from build123d import *

# Parameters (mm, degrees)
SKETCH1_R           = 12.578
SKETCH1_R_2         = 9.398
BOSS_EXTRUDE1_DEPTH = 3.175
FILLET1_R           = 38.1
FILLET2_R           = 6.35


with BuildPart() as part:
    # Sketch1 → Boss-Extrude1 (new, symmetric)
    # profile 1 of 4: a face of its own
    with BuildSketch(Plane.XY):
        with BuildLine():
            Line((550.906377784, 50.55819174), (568.724608053, 41.896435909))
            ThreePointArc((568.724608053, 41.896435909), (571.307203408, 34.427721881), (563.838489379, 31.845126527))
            Line((563.838489379, 31.845126527), (546.02025911, 40.506882357))
            Line((546.02025911, 40.506882357), (543.244055318, 34.795911117))
            Line((543.244055318, 34.795911117), (602.068897859, 6.200118203))
            Line((602.068897859, 6.200118203), (619.322536705, 15.354662769))
            ThreePointArc((619.322536705, 15.354662769), (624.245533427, 18.531839743), (630.07371037, 19.134088663))
            Line((630.07371037, 19.134088663), (553.682581576, 56.26916298))
            Line((553.682581576, 56.26916298), (550.906377784, 50.55819174))
        make_face()
    # profile 2 of 4: a face of its own
    with BuildSketch(Plane.XY):
        with BuildLine():
            ThreePointArc((619.635184113, -2.3391632), (615.840878926, 6.443467165), (619.322536705, 15.354662769))
            Line((619.322536705, 15.354662769), (602.068897859, 6.200118203))
            Line((602.068897859, 6.200118203), (619.635184113, -2.3391632))
        make_face()
    # profile 3 of 4: a face of its own
    with BuildSketch(Plane.XY):
        with Locations((628.416915809, 6.665683962)):
            Circle(SKETCH1_R)
        with Locations((628.416915809, 6.665683962)):
            Circle(SKETCH1_R_2, mode=Mode.SUBTRACT)
    # profile 4 of 4: a face of its own
    with BuildSketch(Plane.XY):
        with BuildLine():
            Line((619.635184113, -2.3391632), (602.068897859, 6.200118203))
            Line((602.068897859, 6.200118203), (544.291028723, -24.456028169))
            Line((544.291028723, -24.456028169), (547.267260579, -30.065354683))
            Line((547.267260579, -30.065354683), (564.768359303, -20.779511294))
            ThreePointArc((564.768359303, -20.779511294), (572.323650668, -23.096634594), (570.006527369, -30.651925959))
            Line((570.006527369, -30.651925959), (552.505428645, -39.937769348))
            Line((552.505428645, -39.937769348), (555.4816605, -45.547095862))
            Line((555.4816605, -45.547095862), (630.513168482, -5.736404924))
            ThreePointArc((630.513168482, -5.736404924), (624.667353131, -5.3404338), (619.635184113, -2.3391632))
        make_face()
    extrude(amount=BOSS_EXTRUDE1_DEPTH, both=True)

    # Fillet1
    # the kernel refuses this fillet: 38.1 mm, written as the material it adds along each edge
    with BuildSketch(Plane(origin=(602.068897859, 6.200118203, -3.175), x_dir=(-0.8993655496308585, 0.43719744754193623, 0), z_dir=(0, 0, 1))) as fillet1_piece_1:
        with BuildLine():
            CenterArc((73.33595186, 37.265834599), FILLET1_R, 155.886500773, 102.102011478)
            Line((38.560636086, 52.831418843), (0, 0))
            Line((0, 0), (65.407044516, 0))
        make_face()
    extrude(amount=6.35)

    # Fillet2
    fillet2_edges = [part.edges().sort_by_distance(p)[0] for p in [
        (630.07371037, 19.134088663, 0),
        (630.513168482, -5.736404924, 0),
    ]]
    fillet(fillet2_edges, radius=FILLET2_R)


solid = part.part
Geometry check sheet. Reference: the model listing, model coordinates, mm. A direction names the side the tool comes from. Give positions to 0.01 mm unless a question says otherwise; leave off trailing zeros. Loops run counter-clockwise (first coordinate to the right, second up) from the corner with the lowest first, then second, coordinate; pieces in that order, holes last. Notation, with made-up numbers: (-36, -21) -> (8, -21) arc R32 ccw to (8, 14) -> close; hole circle Ø11 at (-9.75, -32). An arc over 180 degrees is marked (long way). Answer in a Markdown table with one row per item. Add a question column.
1) Gauge pin test, flat ends, axial feed: P1, Ø1.5, axis at x = 591.5, z = 0.5, coming from the +Y side; P2, Ø1.5, axis at x = 565.5, z = 2, coming from the -Y side; P3, Ø3, axis at x = 573, z = -2, coming from the -Y side. Record the tip position at first contact, or that the pin passes through.
2) Set-up check for faces 4 (the face through (583, 2, 3.175)), 5 (the face through (555.054, 36.115, 0.044)), 6 (the face through (559.69, 46.29, 0.04)): record each of +Z, -Z, +X, -X, +Y, -Y from which the full face is reachable in a straight line by a thin tool's end or side.
3) Cross-section at C-C on z = -1.5. Record the boundary of the cut face in (x, y).
4) Material ranges on probe 1 along Y at (x, z) = (569.5, -1.75); probe 2 along Y at (x, z) = (566.5, -2.75); probe 3 along Y at (x, z) = (628.5, -0.75), recorded low to high. Write a range as from..to.
5) Cross-section at B-B on y = -27. Record the boundary of the cut face in (x, z) (3 decimals).
6) Cross-section at A-A on x = 621. Record the boundary of the cut face in (y, z) (3 decimals).
7) Draft check along Y on faces 1 (the face through (561.38, -35.23, 0.04)), 2 (the face through (553.97, -42.7, 0.04)), 3 (the face through (544.65, 37.69, 0.04)). Enter one of: pulls with the +Y half, pulls with the -Y half, needs draft (parallel to the pull), parting line crosses it, or undercut.
8) Cross-section at D-D on x = 593. Record the boundary of the cut face in (y, z) (3 decimals).
Outcome:
| question | item | result |
|---|---|---|
| 1 | P1 | stops at y = 38.25 |
| 1 | P2 | stops at y = -40.63 |
| 1 | P3 | stops at y = -37.05 |
| 2 | face 4 | +Z, +X, -X, +Y, -Y |
| 2 | face 5 | +Z, -Z |
| 2 | face 6 | +Z, -Z, -X |
| 3 | outline | (543.24, 34.8) arc R38.1 cw to (544.29, -24.46) -> (547.27, -30.07) -> (564.77, -20.78) arc R5.59 cw to (570.01, -30.65) -> (552.51, -39.94) -> (555.48, -45.55) -> (629.7, -6.17) arc R6.35 cw to (631.25, -5.59) arc R12.58 ccw to (630.81, 19.01) arc R6.35 cw to (629.25, 19.54) -> (553.68, 56.27) -> (550.91, 50.56) -> (568.72, 41.9) arc R5.59 cw to (563.84, 31.85) -> (546.02, 40.51) -> close; hole circle Ø18.8 at (628.42, 6.67) |
| 4 | probe 1 | y = -38.11..-30.92, -20.54..32.3, 41.44..48.58 |
| 4 | probe 2 | y = -39.7..-32.51, -20.2..31.29, 42.98..50.04 |
| 4 | probe 3 | y = -6.8..-2.73, 16.06..19.9 |
| 5 | outline | (545.641, -3.175) -> (553.045, -3.175) -> (553.045, 3.175) -> (545.641, 3.175) -> close; (572.826, -3.175) -> (590.438, -3.175) -> (590.438, 3.175) -> (572.826, 3.175) -> close |
| 6 | outline | (-10.784, -3.175) -> (0.894, -3.175) -> (0.894, 3.175) -> (-10.784, 3.175) -> close; (12.437, -3.175) -> (23.545, -3.175) -> (23.545, 3.175) -> (12.437, 3.175) -> close |
| 7 | face 1 | undercut |
| 7 | face 2 | pulls with the -Y half |
| 7 | face 3 | pulls with the +Y half |
| 8 | outline | (-25.64, -3.175) -> (37.156, -3.175) -> (37.156, 3.175) -> (-25.64, 3.175) -> close |
